Part model, mm, in its own coordinate system. Face numbers are marked on the shaded views. Round coordinates to 2 decimals unless told otherwise and drop trailing zeros. Order: outer loops, then holes, each group sorted by start corner. A loop starts at its lowest first (then second) coordinate and runs counter-clockwise, first axis right, second up. Notation, with made-up numbers: (0, 10) -> (33, 10) arc R32 ccw to (33, 40) -> close; hole circle Ø3 at (-21, -6). An arc over 180 degrees is marked (long way). Answer as a JSON object with one key per item and string values. Group by question number.
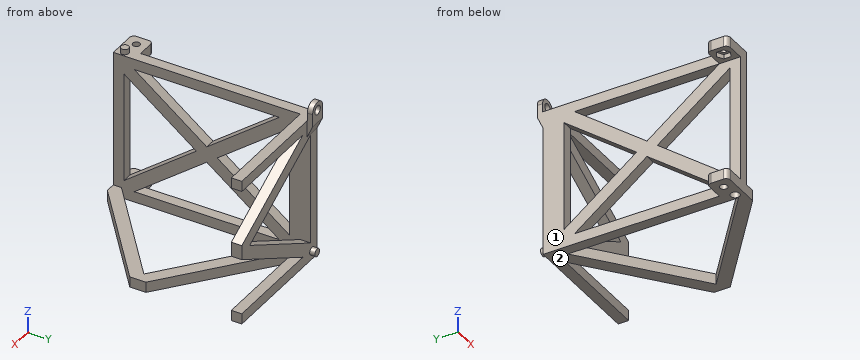
```python
from build123d import *

# Parameters (mm, degrees)
SKETCH_W                   = 55
SKETCH_H                   = 44.5
PAD_DEPTH                  = 5
PAD001_DEPTH               = 5
PAD001_MIRRORED001_2_DEPTH = 5
PAD002_DEPTH               = 5
SKETCH003_R                = 1.85
PAD003_DEPTH               = 2.5
SKETCH004_R                = 2.15
PAD004_DEPTH               = 2.7
SKETCH005_W                = 0.2
SKETCH005_H                = 8
POCKET_DEPTH               = 60.001
SKETCH006_R                = 1.85
PAD005_DEPTH               = 2.5
SKETCH007_R                = 2.15
POCKET001_DEPTH            = 3
PAD006_DEPTH               = 5
SKETCH009_R                = 1.8
HOLE_DEPTH                 = 25
HOLE_TIPS_R                = 1.8
PAD007_DEPTH               = 5
POCKET002_DEPTH            = 2.15
SKETCH012_R                = 1.7
HOLE001_DEPTH              = 10.851
POCKET003_DEPTH            = 290.201912


with BuildPart() as part:
    # Sketch → Pad (new body)
    with BuildSketch(Plane.XY):
        with Locations((-27.5, -22.25)):
            Rectangle(SKETCH_W, SKETCH_H)
    pad = extrude(amount=PAD_DEPTH)

    # Mirrored: Pad across XZ
    add(pad.mirror(Plane.XZ))

    # Sketch001 (on Face1 of Mirrored) → Pad001 (join)
    with BuildSketch(Plane(origin=(-55, 0, 0), x_dir=(0, -1, 0), z_dir=(-1, 0, 0))):
        Polygon((0, 0), (44.5, 0), (44.5, 35), (39.5, 35), (39.5, 8.767158), (4.960091, 35), (0, 35), (0, 31.232842), (34.539909, 5), (0, 5), align=None)
    pad001 = extrude(amount=PAD001_DEPTH)

    # Sketch001 Mirrored001 2 → Pad001 Mirrored001 2 (add)
    with BuildSketch(Plane.YZ.offset(-55)):
        Polygon((0, 0), (44.5, 0), (44.5, 35), (39.5, 35), (39.5, 8.767158), (4.960091, 35), (0, 35), (0, 31.232842), (34.539909, 5), (0, 5), align=None)
    pad001_mirrored001_2 = extrude(amount=-PAD001_MIRRORED001_2_DEPTH)

    # Mirrored002: Pad001, Pad001 Mirrored001 2 across face of Pad001
    add(pad001.mirror(Plane(origin=(-57.5, -2.480045, 35), x_dir=(1, 0, 0), z_dir=(0, 0, 1))))
    add(pad001_mirrored001_2.mirror(Plane(origin=(-57.5, -2.480045, 35), x_dir=(1, 0, 0), z_dir=(0, 0, 1))))

    # Sketch002 (on Face1 of MultiTransform) → Pad002 (join)
    with BuildSketch(Plane(origin=(0, 44.5, 0), x_dir=(-1, 0, 0), z_dir=(0, 1, 0))):
        Polygon((6.264982, 35), (55, 8.417263), (55, 35), (60, 35), (60, 0), (0, 0), (0, 5), (48.735018, 5), (0, 31.582737), (0, 35), align=None)
    pad002 = extrude(amount=PAD002_DEPTH)

    # Mirrored003: Pad002 across face of Pad002
    add(pad002.mirror(Plane(origin=(-3.132491, 47, 35), x_dir=(1, 0, 0), z_dir=(0, 0, 1))))

    # Sketch003 (on Face8 of Mirrored003) → Pad003 (join)
    with BuildSketch(Plane(origin=(0, 49.5, 0), x_dir=(-1, 0, 0), z_dir=(0, 1, 0))):
        with Locations((56, 4)):
            Circle(SKETCH003_R)
    extrude(amount=PAD003_DEPTH)

    # Sketch004 (on Face19 of Pad003) → Pad004 (join)
    with BuildSketch(Plane(origin=(0, 49.5, 0), x_dir=(-1, 0, 0), z_dir=(0, 1, 0))):
        with BuildLine():
            Line((60, 62), (60, 74))
            ThreePointArc((60, 74), (56, 78), (52, 74))
            Line((52, 74), (52, 62))
            Line((52, 62), (60, 62))
        make_face()
        with Locations((56, 74)):
            Circle(SKETCH004_R, mode=Mode.SUBTRACT)
    extrude(amount=PAD004_DEPTH)

    # Sketch005 (on Face56 of Pad004) → Pocket (cut, through all)
    with BuildSketch(Plane(origin=(-60, 0, 0), x_dir=(0, -1, 0), z_dir=(-1, 0, 0))):
        Polygon((-52.2, 68), (-49.5, 62), (-52.2, 62), align=None)
        with Locations((-49.6, 74)):
            Rectangle(SKETCH005_W, SKETCH005_H)
    extrude(amount=-POCKET_DEPTH, mode=Mode.SUBTRACT)

    # Sketch006 (on Face59 of Pocket) → Pad005 (join)
    with BuildSketch(Plane.XY.offset(70)):
        with Locations((-57.5, -40.5)):
            Circle(SKETCH006_R)
    extrude(amount=PAD005_DEPTH)

    # Sketch007 (on Face24 of Pad005) → Pocket001 (cut)
    with BuildSketch(Plane(origin=(0, 0, 0), x_dir=(1, 0, 0), z_dir=(0, 0, -1))):
        with Locations((-57.5, 40.5)):
            Circle(SKETCH007_R)
    extrude(amount=-POCKET001_DEPTH, mode=Mode.SUBTRACT)

    # Sketch008 (on Face24 of Pocket001) → Pad006 (join)
    with BuildSketch(Plane(origin=(0, 0, 0), x_dir=(1, 0, 0), z_dir=(0, 0, -1))):
        with BuildLine():
            Line((-60, 44.5), (-68, 44.5))
            ThreePointArc((-68, 44.5), (-69.414214, 43.914214), (-70, 42.5))
            Line((-70, 42.5), (-70, 39.5))
            Line((-70, 39.5), (-60, 39.5))
            Line((-60, 39.5), (-60, 44.5))
        make_face()
    pad006 = extrude(amount=-PAD006_DEPTH)

    # Mirrored004: Pad006 across face of Pad006
    add(pad006.mirror(Plane(origin=(-65, -39.5, 2.5), x_dir=(-1, 0, 0), z_dir=(0, 1, 0))))

    # Sketch009 (on Face46 of Mirrored004) → Hole (cut)
    with BuildSketch(Plane(origin=(0, 0, 0), x_dir=(1, 0, 0), z_dir=(0, 0, -1))):
        with Locations((-65, 39.5)):
            Circle(SKETCH009_R)
    extrude(amount=-HOLE_DEPTH, mode=Mode.SUBTRACT)

    # Hole tips → Hole tip 1 section 0
    with BuildSketch(Plane(origin=(0, 0, 25), x_dir=(1, 0, 0), z_dir=(0, 0, -1)), mode=Mode.PRIVATE) as hole_tip_1_s0:
        with Locations((-65, 39.5)):
            Circle(HOLE_TIPS_R)
    loft([hole_tip_1_s0.sketch, Vertex(-65, -39.5, 26.081549)], mode=Mode.SUBTRACT)

    # Sketch010 (on Face65 of Hole) → Pad007 (join)
    with BuildSketch(Plane.XY.offset(70)):
        with BuildLine():
            Line((-60, -44.5), (-68, -44.5))
            ThreePointArc((-70, -42.5), (-69.414214, -43.914214), (-68, -44.5))
            Line((-70, -42.5), (-70, -39.5))
            Line((-70, -39.5), (-60, -39.5))
            Line((-60, -39.5), (-60, -44.5))
        make_face()
    pad007 = extrude(amount=-PAD007_DEPTH)

    # Mirrored005: Pad007 across face of Pad007
    add(pad007.mirror(Plane(origin=(-65, -39.5, 67.5), x_dir=(-1, 0, 0), z_dir=(0, 1, 0))))

    # Sketch011 (on Face89 of Mirrored005) → Pocket002 (cut)
    with BuildSketch(Plane(origin=(0, 0, 65), x_dir=(1, 0, 0), z_dir=(0, 0, -1))):
        Polygon((-65, 42.848632), (-67.9, 41.174316), (-67.9, 37.825684), (-65, 36.151368), (-62.1, 37.825684), (-62.1, 41.174316), align=None)
    extrude(amount=-POCKET002_DEPTH, mode=Mode.SUBTRACT)

    # Sketch012 (on Face102 of Pocket002) → Hole001 (cut, through all)
    with BuildSketch(Plane(origin=(0, 0, 67.15), x_dir=(1, 0, 0), z_dir=(0, 0, -1))):
        with Locations((-65, 39.5)):
            Circle(SKETCH012_R)
    extrude(amount=-HOLE001_DEPTH, mode=Mode.SUBTRACT)

    # Sketch013 (on Face11 of Hole001) → Pocket003 (cut, through all)
    with BuildSketch(Plane.XY.offset(5)):
        Polygon((0, -3.85897), (-50.230486, -44.5), (0, -44.5), align=None)
        Polygon((-55, 0), (-4.769514, 0), (-55, -40.64103), align=None)
    pocket003 = extrude(amount=-POCKET003_DEPTH, mode=Mode.SUBTRACT)

    # Mirrored006: Pocket003 across XZ
    add(pocket003.mirror(Plane.XZ), mode=Mode.SUBTRACT)


solid = part.part
```
Q1. Two-plate mould, pull along Z, no slides. Class the marked faces 1 and 2: +Z half, -Z half, draft (parallel to the pull), parting line (faces both ways), or undercut.
Q2. Drop flat-ended pins along their axis: pin 1 Ø4 at (x, z) = (-55.5, 4.5) entering from +Y; pin 2 Ø4 at (x, z) = (-65.5, 2.5) entering from +Y; pin 3 Ø10 at (x, z) = (-63, 32.5) entering from +Y. Give the stop position or say it passes through.
Q3. Band-saw the part on A-A (z = 10.5). List the corners of the cut face in (x, y).
Q4. Wall check: line 1 (Z direction, x = -62, y = -37.5); line 2 (Y direction, x = -57.5, z = 1.15); line 3 (X direction, y = 51, z = 74). Give the ranges that are in metal, low to high. Write a range as [from, to].
Q5. Band-saw the part on C-C (y = 14.5). List the corners of the cut face in (x, z).
Q6. Band-saw the part on B-B (x = -35). List the corners of the cut face in (y, z), plus the area to 3 significant figures.
Completed:
{
 "1": {"face 1": "undercut", "face 2": "-Z half"},
 "2": {"pin 1": "y = 52", "pin 2": "y = -34.5", "pin 3": "y = 49.5"},
 "3": {"outline": "(-60, -44.5) -> (-55, -44.5) -> (-55, -39.5) -> (-60, -39.5) -> close; (-60, -37.22) -> (-55, -37.22) -> (-55, -27.3) -> (-60, -27.3) -> close; (-60, 27.3) -> (-55, 27.3) -> (-55, 37.22) -> (-60, 37.22) -> close; (-60, 39.5) -> (-55, 39.5) -> (-55, 49.5) -> (-60, 49.5) -> close; (-51.18, 44.5) -> (-38.65, 44.5) -> (-38.65, 49.5) -> (-51.18, 49.5) -> close"},
 "4": {"line 1": "[0, 5], [65, 70]", "line 2": "[-44.5, -42.65], [-38.35, 49.5]", "line 3": "[-60, -58.15], [-53.85, -52]"},
 "5": {"outline": "(-60, 0) -> (-55, 0) -> (-55, 5) -> (-60, 5) -> close; (-60, 20.22) -> (-55, 20.22) -> (-55, 27.75) -> (-60, 27.75) -> close; (-60, 42.25) -> (-55, 42.25) -> (-55, 49.78) -> (-60, 49.78) -> close; (-60, 65) -> (-55, 65) -> (-55, 70) -> (-60, 70) -> close; (-22.69, 0) -> (-13.15, 0) -> (-13.15, 5) -> (-22.69, 5) -> close"},
 "6": {"outline": "(-32.18, 0) -> (-24.46, 0) -> (-24.46, 5) -> (-32.18, 5) -> close; (24.46, 0) -> (32.18, 0) -> (32.18, 5) -> (24.46, 5) -> close; (44.5, 0) -> (49.5, 0) -> (49.5, 5) -> (44.5, 5) -> close; (44.5, 12.49) -> (49.5, 12.49) -> (49.5, 19.33) -> (44.5, 19.33) -> close; (44.5, 50.67) -> (49.5, 50.67) -> (49.5, 57.51) -> (44.5, 57.51) -> close; (44.5, 65) -> (49.5, 65) -> (49.5, 70) -> (44.5, 70) -> close", "area": "196 mm2"}
}
